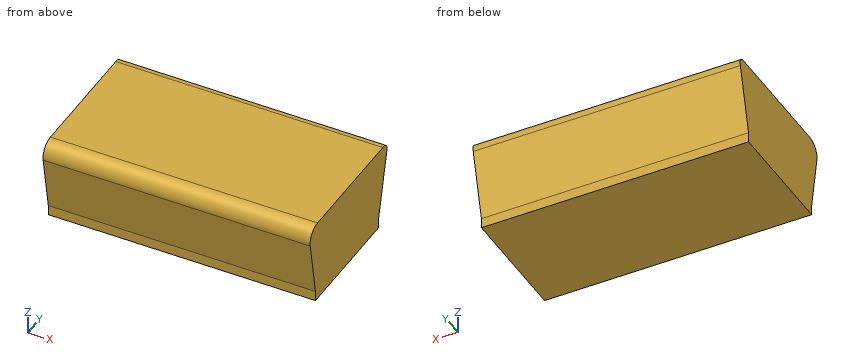
from build123d import *

# Parameters (mm, degrees)
F0_W        = 470
F0_H        = 40
F1_DEPTH    = 1050
F2_R        = 55
F3_T1_DEPTH = 1240.5148333467


# Not quite as in the source:
# - a fillet or chamfer that OpenCascade refuses, or shapes differently, is made with other operations: its cross-section is extruded or revolved along the edge and cut away or added


with BuildPart() as f1:
    # F0 (on Right) → F1 (new body)
    with BuildSketch(Plane.YZ):
        Polygon((-50, 290), (0, 0), (470, 0), (540, 290), (470, 290), align=None)
        with Locations((235, -20)):
            Rectangle(F0_W, F0_H)
    extrude(amount=F1_DEPTH)

    # F2
    f2_edges = [f1.edges().sort_by_distance(p)[0] for p in [
        (525, -50, 290),
    ]]
    fillet(f2_edges, radius=F2_R)

    # F3: fillet of radius 30 on 1 edges, made by hand

    # F3_s2 → F3_t1 (cut)
    with BuildSketch(Plane.YZ.offset(-95.2574166733)):
        with BuildLine():
            add(Edge.make_bspline(
                [(501.8970333307, 290), (540, 290), (531.0594995879, 252.9607840069)],
                knots=[0, 0, 0, 1, 1, 1], degree=2, weights=[1, 1, 1]))
            Line((531.0594995879, 252.9607840069), (540, 290))
            Line((540, 290), (501.8970333307, 290))
        make_face()
    extrude(amount=F3_T1_DEPTH, mode=Mode.SUBTRACT)


solid = f1.part
Work out the finished part from the listing and answer in its coordinate system (mm). Round coordinates to 2 decimals unless told otherwise and drop trailing zeros. Write each loop counter-clockwise with the first axis right and the second up, starting at its lowest first coordinate (ties: lowest second). Pieces come first, ordered by that corner, then holes.
1) Given pin 1 Ø12 at (x, z) = (892.5, 13.5) entering from -Y; pin 2 Ø4 at (x, z) = (913, 8) entering from -Y; pin 3 Ø12 at (x, z) = (132, 216.5) entering from +Y, each flat-ended and moving along its own axis, determine where each tip first touches the part or whether it passes through.
2) A cutting plane is placed at B-B (z = 43). Give the vertices of the cut face in (x, y), plus the area to 3 significant figures.
3) Straight lines are drawn through the part: line 1 (Y direction, x = 456, z = -19.5); line 2 (Y direction, x = 433.5, z = 189.5). For each, find the intervals that lie inside material, in ascending order.
4) A cutting plane is placed at A-A (z = -12). Give the vertices of the cut face in (x, y).
Completed:
1. pin 1: stops at y = -3.36
1. pin 2: stops at y = -1.72
1. pin 3: stops at y = 523.71
2. outline: (0, -7.41) - (1050, -7.41) - (1050, 480.38) - (0, 480.38) - close
2. area: 512,000 mm2
3. line 1: y = 0 to 470
3. line 2: y = -32.67 to 515.74
4. outline: (0, 0) - (1050, 0) - (1050, 470) - (0, 470) - close
